Part model, mm, in its own coordinate system. Give positions to 0.01 mm unless a question says otherwise; leave off trailing zeros. Order: outer loops, then holes, each group sorted by start corner. A loop starts at its lowest first (then second) coordinate and runs counter-clockwise, first axis right, second up. Notation, with made-up numbers: (-35, 75) -> (-20, 75) arc R18 cw to (-20, 80) -> close; hole circle Ø8 at (2, 47.25). An arc over 180 degrees is marked (long way). Write item = value, one per line. Start each with the question number.
Item 1: Pull direction Y, two halves, no side cores. Call faces 1 (the face through (-1.11, 16.01, 1.48)), 2 (the face through (-2, 15, 3)), 3 (the face through (0, 37, 1)): +Y half, -Y half, draft (parallel to the pull), parting line (faces both ways), or undercut.
Item 2: Band-saw the part on A-A on y = 15. Write the cut outline in (x, z), plus the area to 3 significant figures.
Item 3: Band-saw the part on B-B on x = 2.75. Write the cut outline in (y, z), plus the area to 3 significant figures.
Item 4: Band-saw the part on D-D on x = 0. Write the cut outline in (y, z), plus the area to 3 significant figures.
Item 5: Flat gauge pins, fed straight in: P1, Ø6.5, axis at x = 0, y = 30, coming from the -Z side; P2, Ø1, axis at x = 5, z = 1, coming from the +Y side; P3, Ø8, axis at x = -3.5, y = -0.5, coming from the +Z side; P4, Ø1.5, axis at x = 2.5, z = 1.5, coming from the +Y side. Where does each tip first touch, or does it go through?
Item 6: Drill centre lines: line 1 along Y through (x, z) = (0, 1.5); line 2 along Y through (x, z) = (-3.5, 0.8); line 3 along Y through (x, z) = (-1.25, 0.5). Where is each one in solid material? Low to high.
Item 7: Band-saw the part on C-C on z = 2.35. Write the cut outline in (x, y).
```python
from build123d import *

# Parameters (mm, degrees)
SKETCH_1_R      = 7
SKETCH_1_R_2    = 3.95
SKETCH_1_R_3    = 1.5
EXTRUDE_1_DEPTH = 3


with BuildPart() as part:
    # 草图1 → 凸台-拉伸1 (new body)
    # profile 1 of 3: a face of its own
    with BuildSketch(Plane.XY):
        with Locations((0, 30)):
            Circle(SKETCH_1_R)
        with Locations((0, 30)):
            Circle(SKETCH_1_R_2, mode=Mode.SUBTRACT)
    # profile 2 of 3: a face of its own
    with BuildSketch(Plane.XY):
        with BuildLine():
            ThreePointArc((7, 30), (0, 23), (-7, 30))
            Line((-7, 30), (-7, 0))
            ThreePointArc((-7, 0), (0, 7), (7, 0))
            Line((7, 0), (7, 30))
        make_face()
        with Locations((0, 15)):
            Circle(SKETCH_1_R_3, mode=Mode.SUBTRACT)
    # profile 3 of 3: a face of its own
    with BuildSketch(Plane.XY):
        Circle(SKETCH_1_R)
        Circle(SKETCH_1_R_2, mode=Mode.SUBTRACT)
    extrude(amount=EXTRUDE_1_DEPTH)


solid = part.part
```
Values found:
q1.face_1 = undercut
q1.face_2 = draft
q1.face_3 = +Y half
q2.outline = (-7, 0) -> (-1.5, 0) -> (-1.5, 3) -> (-7, 3) -> close; (1.5, 0) -> (7, 0) -> (7, 3) -> (1.5, 3) -> close
q2.area = 33.0 mm^2
q3.outline = (-6.44, 0) -> (-2.84, 0) -> (-2.84, 3) -> (-6.44, 3) -> close; (2.84, 0) -> (27.16, 0) -> (27.16, 3) -> (2.84, 3) -> close; (32.84, 0) -> (36.44, 0) -> (36.44, 3) -> (32.84, 3) -> close
q3.area = 94.6 mm^2
q4.outline = (-7, 0) -> (-3.95, 0) -> (-3.95, 3) -> (-7, 3) -> close; (3.95, 0) -> (13.5, 0) -> (13.5, 3) -> (3.95, 3) -> close; (16.5, 0) -> (26.05, 0) -> (26.05, 3) -> (16.5, 3) -> close; (33.95, 0) -> (37, 0) -> (37, 3) -> (33.95, 3) -> close
q4.area = 75.6 mm^2
q5.P1 = through
q5.P2 = 35.36
q5.P3 = 3
q5.P4 = 36.78
q6.line_1 = -7 to -3.95, 3.95 to 13.5, 16.5 to 26.05, 33.95 to 37
q6.line_2 = -6.06 to -1.83, 1.83 to 28.17, 31.83 to 36.06
q6.line_3 = -6.89 to -3.75, 3.75 to 14.17, 15.83 to 26.25, 33.75 to 36.89
q7.outline = (-7, 0) arc R7 ccw to (7, 0) -> (7, 30) arc R7 ccw to (-7, 30) -> close; hole circle Ø7.9 at (0, 0); hole circle Ø7.9 at (0, 30); hole circle Ø3 at (0, 15)
